```python
from build123d import *

# Parameters (mm, degrees)
SKETCH1_R           = 40
BOSS_EXTRUDE1_DEPTH = 10
BOSS_EXTRUDE6_DEPTH = 5
BOSS_EXTRUDE7_START = -15
BOSS_EXTRUDE7_DEPTH = 5


with BuildPart() as part:
    # Sketch1 → Boss-Extrude1 (new body)
    with BuildSketch(Plane(origin=(0, 0, 0), x_dir=(1, 0, 0), z_dir=(0, 1, 0))):
        with Locations(Location((0, 0, 0), (0, 0, 270))):
            Circle(SKETCH1_R)
        with BuildLine():
            Line((-2, 23.665639649), (-0.800587161, 26.237788783))
            ThreePointArc((-0.800587161, 26.237788783), (0, 26.25), (0.800587161, 26.237788783))
            Line((0.800587161, 26.237788783), (2, 23.665639649))
            ThreePointArc((2, 23.665639649), (11.875, 20.56810334), (19.495045133, 13.564870632))
            Line((19.495045133, 13.564870632), (22.322298044, 13.812223211))
            ThreePointArc((22.322298044, 13.812223211), (22.733166849, 13.125), (23.122885205, 12.425565572))
            Line((23.122885205, 12.425565572), (21.495045133, 10.100769017))
            ThreePointArc((21.495045133, 10.100769017), (23.75, 0), (21.495045133, -10.100769017))
            Line((21.495045133, -10.100769017), (23.122885205, -12.425565572))
            ThreePointArc((23.122885205, -12.425565572), (22.733166849, -13.125), (22.322298044, -13.812223211))
            Line((22.322298044, -13.812223211), (19.495045133, -13.564870632))
            ThreePointArc((19.495045133, -13.564870632), (11.875, -20.56810334), (2, -23.665639649))
            Line((2, -23.665639649), (0.800587161, -26.237788783))
            ThreePointArc((0.800587161, -26.237788783), (0, -26.25), (-0.800587161, -26.237788783))
            Line((-0.800587161, -26.237788783), (-2, -23.665639649))
            ThreePointArc((-2, -23.665639649), (-11.875, -20.56810334), (-19.495045133, -13.564870632))
            Line((-19.495045133, -13.564870632), (-22.322298044, -13.812223211))
            ThreePointArc((-22.322298044, -13.812223211), (-22.733166849, -13.125), (-23.122885205, -12.425565572))
            Line((-23.122885205, -12.425565572), (-21.495045133, -10.100769017))
            ThreePointArc((-21.495045133, -10.100769017), (-23.75, 0), (-21.495045133, 10.100769017))
            Line((-21.495045133, 10.100769017), (-23.122885205, 12.425565572))
            ThreePointArc((-23.122885205, 12.425565572), (-22.733166849, 13.125), (-22.322298044, 13.812223211))
            Line((-22.322298044, 13.812223211), (-19.495045133, 13.564870632))
            ThreePointArc((-19.495045133, 13.564870632), (-11.875, 20.56810334), (-2, 23.665639649))
        make_face(mode=Mode.SUBTRACT)
    extrude(amount=BOSS_EXTRUDE1_DEPTH)

    # 4,5,6 → Boss-Extrude6 (add)
    with BuildSketch(Plane(origin=(0, 10, 0), x_dir=(1, 0, 0), z_dir=(0, 1, 0))):
        with BuildLine():
            Line((2.5, 28.892040426), (1.010456949, 32.984526323))
            ThreePointArc((1.010456949, 32.984526323), (0, 33), (-1.010456949, 32.984526323))
            Line((-1.010456949, 32.984526323), (-2.5, 28.892040426))
            ThreePointArc((-2.5, 28.892040426), (0, 29), (2.5, 28.892040426))
        make_face()
        with BuildLine():
            Line((23.771240976, 16.611083723), (28.060209253, 17.367344549))
            ThreePointArc((28.060209253, 17.367344549), (28.578838325, 16.5), (29.070666202, 15.617181774))
            Line((29.070666202, 15.617181774), (26.271240976, 12.280956704))
            ThreePointArc((26.271240976, 12.280956704), (25.11473671, 14.5), (23.771240976, 16.611083723))
        make_face()
        with BuildLine():
            Line((26.271240976, -12.280956704), (29.070666202, -15.617181774))
            ThreePointArc((29.070666202, -15.617181774), (28.578838325, -16.5), (28.060209253, -17.367344549))
            Line((28.060209253, -17.367344549), (23.771240976, -16.611083723))
            ThreePointArc((23.771240976, -16.611083723), (25.11473671, -14.5), (26.271240976, -12.280956704))
        make_face()
        with BuildLine():
            Line((2.5, -28.892040426), (1.010456949, -32.984526323))
            ThreePointArc((1.010456949, -32.984526323), (0, -33), (-1.010456949, -32.984526323))
            Line((-1.010456949, -32.984526323), (-2.5, -28.892040426))
            ThreePointArc((-2.5, -28.892040426), (0, -29), (2.5, -28.892040426))
        make_face()
        with BuildLine():
            Line((-23.771240976, -16.611083723), (-28.060209253, -17.367344549))
            ThreePointArc((-28.060209253, -17.367344549), (-28.578838325, -16.5), (-29.070666202, -15.617181774))
            Line((-29.070666202, -15.617181774), (-26.271240976, -12.280956704))
            ThreePointArc((-26.271240976, -12.280956704), (-25.11473671, -14.5), (-23.771240976, -16.611083723))
        make_face()
        with BuildLine():
            Line((-26.271240976, 12.280956704), (-29.070666202, 15.617181774))
            ThreePointArc((-29.070666202, 15.617181774), (-28.578838325, 16.5), (-28.060209253, 17.367344549))
            Line((-28.060209253, 17.367344549), (-23.771240976, 16.611083723))
            ThreePointArc((-23.771240976, 16.611083723), (-25.11473671, 14.5), (-26.271240976, 12.280956704))
        make_face()
    extrude(amount=BOSS_EXTRUDE6_DEPTH)

    # 4,5,6<2> → Boss-Extrude7 (add)
    with BuildSketch(Plane(origin=(0, 10, 0), x_dir=(1, 0, 0), z_dir=(0, 1, 0)).offset(BOSS_EXTRUDE7_START)):
        with BuildLine():
            Line((2.5, 28.892040426), (1.010456949, 32.984526323))
            ThreePointArc((1.010456949, 32.984526323), (0, 33), (-1.010456949, 32.984526323))
            Line((-1.010456949, 32.984526323), (-2.5, 28.892040426))
            ThreePointArc((-2.5, 28.892040426), (0, 29), (2.5, 28.892040426))
        make_face()
        with BuildLine():
            Line((23.771240976, 16.611083723), (28.060209253, 17.367344549))
            ThreePointArc((28.060209253, 17.367344549), (28.578838325, 16.5), (29.070666202, 15.617181774))
            Line((29.070666202, 15.617181774), (26.271240976, 12.280956704))
            ThreePointArc((26.271240976, 12.280956704), (25.11473671, 14.5), (23.771240976, 16.611083723))
        make_face()
        with BuildLine():
            Line((26.271240976, -12.280956704), (29.070666202, -15.617181774))
            ThreePointArc((29.070666202, -15.617181774), (28.578838325, -16.5), (28.060209253, -17.367344549))
            Line((28.060209253, -17.367344549), (23.771240976, -16.611083723))
            ThreePointArc((23.771240976, -16.611083723), (25.11473671, -14.5), (26.271240976, -12.280956704))
        make_face()
        with BuildLine():
            Line((2.5, -28.892040426), (1.010456949, -32.984526323))
            ThreePointArc((1.010456949, -32.984526323), (0, -33), (-1.010456949, -32.984526323))
            Line((-1.010456949, -32.984526323), (-2.5, -28.892040426))
            ThreePointArc((-2.5, -28.892040426), (0, -29), (2.5, -28.892040426))
        make_face()
        with BuildLine():
            Line((-23.771240976, -16.611083723), (-28.060209253, -17.367344549))
            ThreePointArc((-28.060209253, -17.367344549), (-28.578838325, -16.5), (-29.070666202, -15.617181774))
            Line((-29.070666202, -15.617181774), (-26.271240976, -12.280956704))
            ThreePointArc((-26.271240976, -12.280956704), (-25.11473671, -14.5), (-23.771240976, -16.611083723))
        make_face()
        with BuildLine():
            Line((-26.271240976, 12.280956704), (-29.070666202, 15.617181774))
            ThreePointArc((-29.070666202, 15.617181774), (-28.578838325, 16.5), (-28.060209253, 17.367344549))
            Line((-28.060209253, 17.367344549), (-23.771240976, 16.611083723))
            ThreePointArc((-23.771240976, 16.611083723), (-25.11473671, 14.5), (-26.271240976, 12.280956704))
        make_face()
    extrude(amount=BOSS_EXTRUDE7_DEPTH)


solid = part.part
```
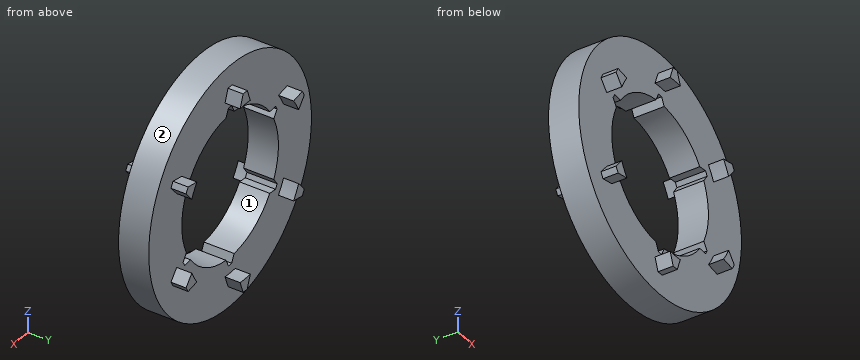
Geometry check sheet. Reference: the model listing, model coordinates, mm. Face numbers are marked on the shaded views. Round coordinates to 2 decimals unless told otherwise and drop trailing zeros. Loops run counter-clockwise (first coordinate to the right, second up) from the corner with the lowest first, then second, coordinate; pieces in that order, holes last. Notation, with made-up numbers: (-27, 47.5) - (28, 47.5) arc R15 ccw to (28, 60.5) - close; hole circle Ø7 at (-17.75, -12.75). An arc over 180 degrees is marked (long way). Use a Markdown table: item, result.
Q1. Cross-section at B-B on x = -11. Record the cut outline in (y, z), plus the area to 3 significant figures.
Solutions:
| item | result |
|---|---|
| outline | (0, -38.46) - (10, -38.46) - (10, -21.05) - (0, -21.05) - close; (0, 21.05) - (10, 21.05) - (10, 38.46) - (0, 38.46) - close |
| area | 348 mm2 |
Q2. Cross-section at A-A on z = 0. Record the cut outline in (x, y).
Solutions:
| item | result |
|---|---|
| outline | (-40, 0) - (-23.75, 0) - (-23.75, 10) - (-40, 10) - close; (23.75, 0) - (40, 0) - (40, 10) - (23.75, 10) - close |
Q3. Draft check along X on the marked faces 1 and 2. Enter one of: released by +X, released by -X, zero draft, split by the parting line, or undercut.
Solutions:
| item | result |
|---|---|
| face 1 | undercut |
| face 2 | split by the parting line |
Q4. Material ranges on line 1 (Y direction, x = -8.5, z = -23.5); line 2 (X direction, y = 7.5, z = -2); line 3 (X direction, y = 4.25, z = -5), recorded low to high.
Solutions:
| item | result |
|---|---|
| line 1 | y = 0 to 10 |
| line 2 | x = -39.95 to -23.67, 23.67 to 39.95 |
| line 3 | x = -39.69 to -23.22, 23.22 to 39.69 |
Q5. Cross-section at C-C on y = 6.25. Record the cut outline in (x, z).
Solutions:
| item | result |
|---|---|
| outline | circle Ø80 at (0, 0); hole (-23.12, -12.43) arc R26.25 ccw to (-22.32, -13.81) - (-19.5, -13.56) arc R23.75 ccw to (-2, -23.67) - (-0.8, -26.24) arc R26.25 ccw to (0.8, -26.24) - (2, -23.67) arc R23.75 ccw to (19.5, -13.56) - (22.32, -13.81) arc R26.25 ccw to (23.12, -12.43) - (21.5, -10.1) arc R23.75 ccw to (21.5, 10.1) - (23.12, 12.43) arc R26.25 ccw to (22.32, 13.81) - (19.5, 13.56) arc R23.75 ccw to (2, 23.67) - (0.8, 26.24) arc R26.25 ccw to (-0.8, 26.24) - (-2, 23.67) arc R23.75 ccw to (-19.5, 13.56) - (-22.32, 13.81) arc R26.25 ccw to (-23.12, 12.43) - (-21.5, 10.1) arc R23.75 ccw to (-21.5, -10.1) - close |
Q6. Go/stop test with flat-tipped pins: P1, Ø10, axis at x = 8, y = 9, coming from the -Z side; P2, Ø3, axis at x = -19, z = -19.5, coming from the -Y side; P3, Ø8, axis at x = -6, z = 23, coming from the +Y side. Record where each tip stops, or that it passes through.
Solutions:
| item | result |
|---|---|
| P1 | stops at z = -39.89 |
| P2 | stops at y = 0 |
| P3 | stops at y = 10 |
